Geometry: final body of the model. Coordinates: model frame, mm. A direction names the side the tool comes from. Coordinates: 2 decimals unless noted, no trailing zeros. Order: outer loops, then holes, each group sorted by start corner. A loop starts at its lowest first (then second) coordinate and runs counter-clockwise, first axis right, second up. Notation, with made-up numbers: M -29,79 L 20,79 A21 ccw 20,90 Z; hole C -3,-11.5 d2. An arc over 180 degrees is marked long. One line per question, with ' | ' between items.
from build123d import *

# Parameters (mm, degrees)
F0_W     = 44.45
F0_H     = 25.4
F1_DEPTH = 25.4
F2_T     = -2.54
F4_D     = 3.175
F6_D     = 3.175


with BuildPart() as f1:
    # F0 (on Top) → F1 (new body)
    with BuildSketch(Plane.XY):
        with Locations((-7.5998026878, -20.9200205722)):
            Rectangle(F0_W, F0_H)
    extrude(amount=F1_DEPTH)

    # F2
    f2_openings = [f1.faces().sort_by_distance(p)[0] for p in [
        (14.625197, -20.920021, 12.7),
        (-29.824803, -20.920021, 12.7),
        (-7.599803, -33.620021, 12.7),
        (-7.599803, -20.920021, 0),
    ]]
    offset(amount=F2_T, openings=f2_openings)

    # F4 (through all)
    with Locations(Plane(origin=(0, 0, 0), x_dir=(1, 0, 0), z_dir=(0, 1, 0))):
        with Locations((-12.8914693544, -16.9946048409), (-21.3581360211, -16.9946048409)):
            Hole(F4_D / 2)

    # F6 (through all)
    with Locations(Plane.XY.offset(25.4)):
        with Locations((-17.1248026878, -18.3800205722), (1.9251973122, -18.3800205722)):
            Hole(F6_D / 2)


solid = f1.part
1. Material intervals for line 1 (Y direction, x = -7.5, z = 1.5); line 2 (Z direction, x = -1.5, y = -19.75), sorted ascending. Write a range as [from, to].
Response values:
line 1: y = [-10.76, -8.22] | line 2: z = [22.86, 25.4]
2. Draft query along Z for faces 3 (the face through (-12.68, -9.51, 15.42)), 4 (the face through (-8, -33.62, 24)), 5 (the face through (-8, -21, 25.4)), 6 (the face through (-22.212, -9.508, 15.656)). Return one class per face: pulls with the +Z half, pulls with the -Z half, needs draft (parallel to the pull), parting line crosses it, or undercut.
Response values:
face 3: undercut | face 4: needs draft | face 5: pulls with the +Z half | face 6: undercut
3. Section C-C, the plane x = 1. Output: boundary loops of the cut face in (y, z), and give its area (3 significant figures).
Response values:
outline: M -33.62,22.86 L -19.67,22.86 L -19.67,25.4 L -33.62,25.4 Z; M -17.09,22.86 L -10.76,22.86 L -10.76,0 L -8.22,0 L -8.22,25.4 L -17.09,25.4 Z | area: 116 mm^2
4. Section A-A, the plane x = 8. Output: boundary loops of the cut face in (y, z).
Response values:
outline: M -33.62,22.86 L -10.76,22.86 L -10.76,0 L -8.22,0 L -8.22,25.4 L -33.62,25.4 Z
5. Section D-D, the plane z = 20.5. Output: boundary loops of the cut face in (x, y).
Response values:
outline: M -29.82,-10.76 L 14.63,-10.76 L 14.63,-8.22 L -29.82,-8.22 Z
6. Section B-B, the plane z = 17.5. Output: boundary loops of the cut face in (x, y).
Response values:
outline: M -29.82,-10.76 L -22.86,-10.76 L -22.86,-8.22 L -29.82,-8.22 Z; M -19.85,-10.76 L -14.4,-10.76 L -14.4,-8.22 L -19.85,-8.22 Z; M -11.39,-10.76 L 14.63,-10.76 L 14.63,-8.22 L -11.39,-8.22 Z
7. Access query for faces 1 (the face through (-8, -22, 22.86)), 2 (the face through (-16.78, -19.93, 24.11)). Directions: +Z, -Z, +X, -X, +Y, -Y. A direction counts if a zero-diameter tool reaches every point of the face in a straight line with its end or side. Return the directions, or none.
Response values:
face 1: -Z, +X, -X, -Y | face 2: +Z, -Z
8. Pin query (flat end, axial travel): P1, Ø3, axis at x = -10, y = -24, coming from the -Z side; P2, Ø2, axis at x = -23, z = 16, coming from the -Y side; P3, Ø5, axis at x = -8, z = 21, coming from the -Y side. Return the tip coordinate at first contact, or that it passes through.
Response values:
P1: stops at z = 22.86 | P2: stops at y = -10.76 | P3: stops at y = -33.62
